Drawing for the job (mm, zero at the part's lowest x, y, z). A direction names the side the tool comes from. Round coordinates to 2 decimals unless told otherwise and drop trailing zeros. Write each loop counter-clockwise with the first axis right and the second up, starting at its lowest first coordinate (ties: lowest second). Pieces come first, ordered by that corner, then holes. Notation, with made-up numbers: M -24,9 L 3,9 A32 cw 3,39 Z; hole C 43,30 d11. An arc over 180 degrees is marked long. Use a Markdown table: item, result. Add a question column.
1) Slice it at B-B on y = 8. Write the cut outline in (x, z) (1 decimal).
2) Two-plate mould, pull along Y, no slides. Class the marked faces 1, 2, 3 and 4: released by +Y, released by -Y, zero draft, split by the parting line, or undercut.
3) Which spindle directions (+Z, -Z, +X, -X, +Y, -Y) get a long thin tool onto all of the face, cutting with end or side? Do the marked faces 5, 6 and 7. Say none if no direction does.
4) Wall check: probe 1 along Z at (x, y) = (11, 9.75); probe 2 along Z at (x, y) = (9.5, 9.75); probe 3 along Z at (x, y) = (13.5, 8.75). Give the ranges that are in metal, low to high.
5) Slice it at D-D on z = 29. Write the cut outline in (x, y).
6) Slice it at C-C on z = 6. Write the cut outline in (x, y).
7) Slice it at A-A on x = 7.5. Write the cut outline in (y, z).
8) Drop flat-ended pins along their axis: P1, Ø5, axis at x = 12.5, z = 8.5, coming from the +Y side; P2, Ø1, axis at x = 2.5, z = 14.5, coming from the +Y side; P3, Ø2, axis at y = 4.5, z = 13.5, coming from the -X side. Give the stop position or say it passes through.
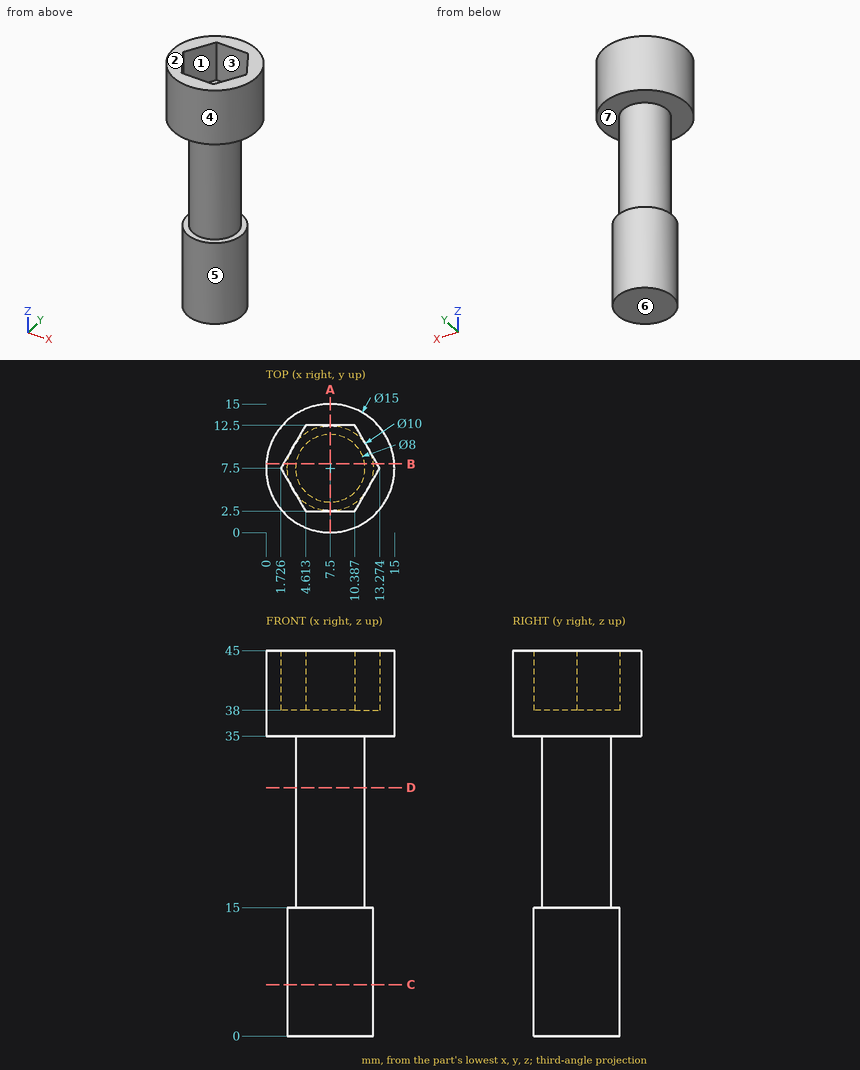
Entries:
| question | item | result |
|---|---|---|
| 1 | outline | M 0,35 L 3.5,35 L 3.5,15 L 2.5,15 L 2.5,0 L 12.5,0 L 12.5,15 L 11.5,15 L 11.5,35 L 15,35 L 15,45 L 13,45 L 13,38 L 2,38 L 2,45 L 0,45 Z |
| 2 | face 1 | undercut |
| 2 | face 2 | zero draft |
| 2 | face 3 | undercut |
| 2 | face 4 | split by the parting line |
| 3 | face 5 | -Z |
| 3 | face 6 | -Z, +X, -X, +Y, -Y |
| 3 | face 7 | none |
| 4 | probe 1 | z = 0 to 15, 35 to 38 |
| 4 | probe 2 | z = 0 to 38 |
| 4 | probe 3 | z = 35 to 45 |
| 5 | outline | C 7.5,7.5 d8 |
| 6 | outline | C 7.5,7.5 d10 |
| 7 | outline | M 0,35 L 3.5,35 L 3.5,15 L 2.5,15 L 2.5,0 L 12.5,0 L 12.5,15 L 11.5,15 L 11.5,35 L 15,35 L 15,45 L 12.5,45 L 12.5,38 L 2.5,38 L 2.5,45 L 0,45 Z |
| 8 | P1 | stops at y = 11.83 |
| 8 | P2 | stops at y = 9.68 |
| 8 | P3 | stops at x = 2.92 |
